Here's the drawing with two shaded views (mm, measured from the low corner). I have some questions. A direction names the side the tool comes from. Coordinates: 2 decimals unless noted, no trailing zeros. Write each loop counter-clockwise with the first axis right and the second up, starting at its lowest first coordinate (ties: lowest second). Pieces come first, ordered by that corner, then holes. Notation, with made-up numbers: (74.25, 20.25) -> (119.25, 20.25) arc R17 ccw to (119.25, 28.25) -> close; hole circle Ø10 at (87.25, 40). An arc over 180 degrees is marked (long way). Put each result on its own line as item: value. Start each with the question number.
Item 1: I want a section at D-D, the plane x = 74. List the corners of the cut face in (y, z) for me, then the cut area to 3 significant figures.
Item 2: I need wall thicknesses on line 1 (X direction, y = 37, z = 29) (1 decimal); line 2 (Y direction, x = 104, z = 59); line 3 (Y direction, x = 127.5, z = 96) (1 decimal). Which ranges of each line are inside material? Lowest first, please. Write a range as [from, to].
Item 3: I want a section at C-C, the plane y = 26. List the corners of the cut face in (x, z) for me (1 decimal), then the cut area to 3 significant figures.
Item 4: I want a section at B-B, the plane z = 105. List the corners of the cut face in (x, y) for me (1 decimal), then the cut area to 3 significant figures.
Item 5: On a 3-axis mill with a long thin cutter (end or side, diameter ignored), from which of +Z, -Z, +X, -X, +Y, -Y can I reach the whole of each face in a straight line? I mean the marked faces 5 and 6. Say none if no direction works.
Item 6: For pin 1 (1 mm diameter, centred on x = 40, z = 45, fed in from +Y), with a flat end and sliding along its axis, tell me the tip position at first contact or that it passes through.
Item 7: If we mould it in two halves opening along Z, with no side actions, what happens to the marked faces 1, 2, 3 and 4? For each: released by +Z, released by -Z, zero draft, split by the parting line, or undercut.
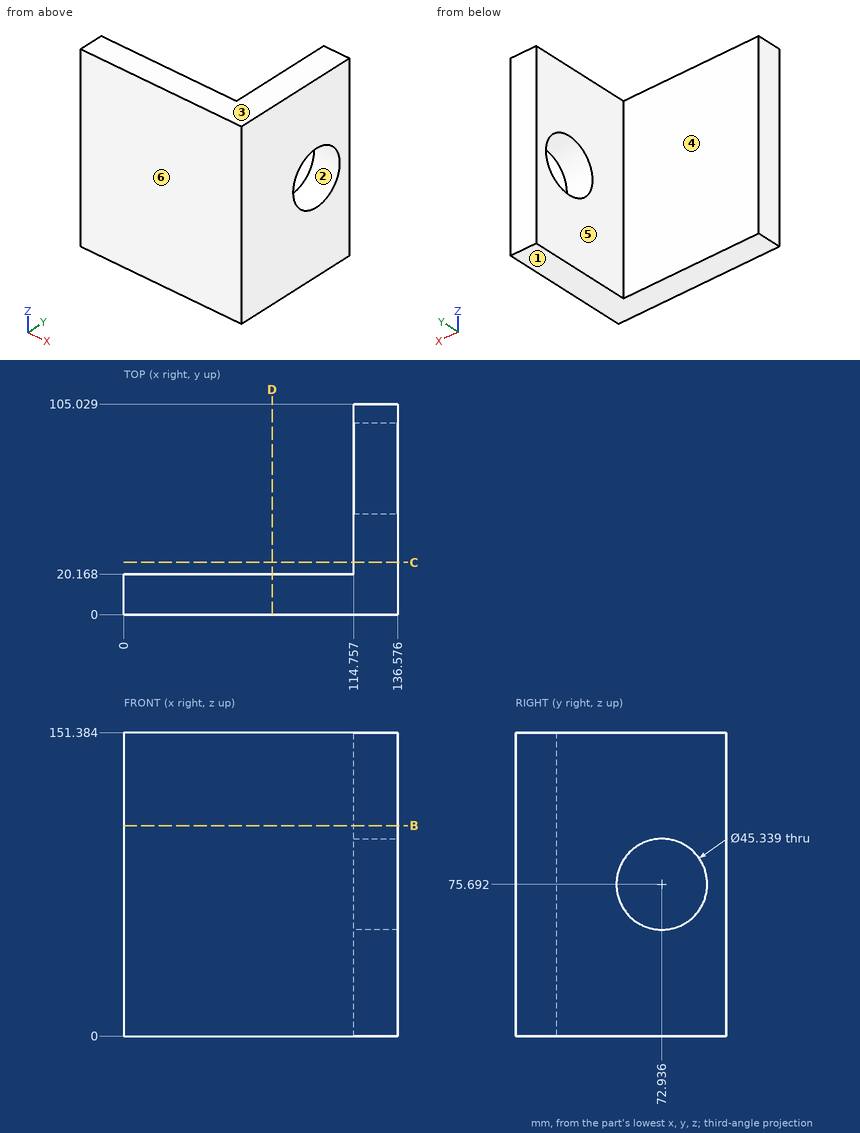
Calculated:
1. outline: (0, 0) -> (20.17, 0) -> (20.17, 151.38) -> (0, 151.38) -> close
1. area: 3,050 mm2
2. line 1: x = [114.8, 136.6]
2. line 2: y = [0, 20.17]
2. line 3: y = [0, 62.9], [83, 105]
3. outline: (114.8, 0) -> (136.6, 0) -> (136.6, 151.4) -> (114.8, 151.4) -> close
3. area: 3,300 mm2
4. outline: (0, 0) -> (136.6, 0) -> (136.6, 105) -> (114.8, 105) -> (114.8, 20.2) -> (0, 20.2) -> close
4. area: 4,610 mm2
5. face 5: +Z, -Z, -X, +Y
5. face 6: +Z, -Z, +X, -X, -Y
6. pin 1: stops at y = 20.17
7. face 1: released by -Z
7. face 2: undercut
7. face 3: released by +Z
7. face 4: zero draft
